The figure shows three views and two pictorial views of one solid part (mm, origin at its lowest corner). Answer the questions. Round coordinates to 2 decimals unless told otherwise and drop trailing zeros. Order: outer loops, then holes, each group sorted by start corner. A loop starts at its lowest first (then second) coordinate and runs counter-clockwise, first axis right, second up. Notation, with made-up numbers: (77.25, 56) -> (82.25, 56) arc R21 ccw to (82.25, 63) -> close; hole circle Ø1 at (-0.5, -0.75). An arc over 180 degrees is marked (long way). Return JSON: item names as keys, results as strings. Group by question number.
(1) The part is cut by section A-A (y = 2). Determine the outline of the cut face in (x, z).
(2) Determine the mould class of the marked faces 1, 2 and 3 for opening direction X: +X half, -X half, draft (parallel to the pull), parting line (faces both ways), or undercut.
(3) Each of these flat-tipped pins is pushed along its axis until it touches: pin 1 (4 mm diameter, centred on x = 17, z = 12, fed in from -Y); pin 2 (4 mm diameter, centred on y = 3, z = 13, fed in from +X). Where does it stop, or does it pass through?
(4) The part is cut by section C-C (z = 13.5). Determine the outline of the cut face in (x, y).
(5) The part is cut by section B-B (x = 50). Determine the outline of the cut face in (y, z) (1 decimal), plus the area to 3 significant figures.
(6) Consider line 1 (X direction, y = 9.75, z = 7.62); line 2 (Z direction, x = 45.72, y = 9.25); line 3 (Z direction, x = 44.5, y = 1.5). Determine where each line is inside the solid, lowest interval first. Write a range as [from, to].
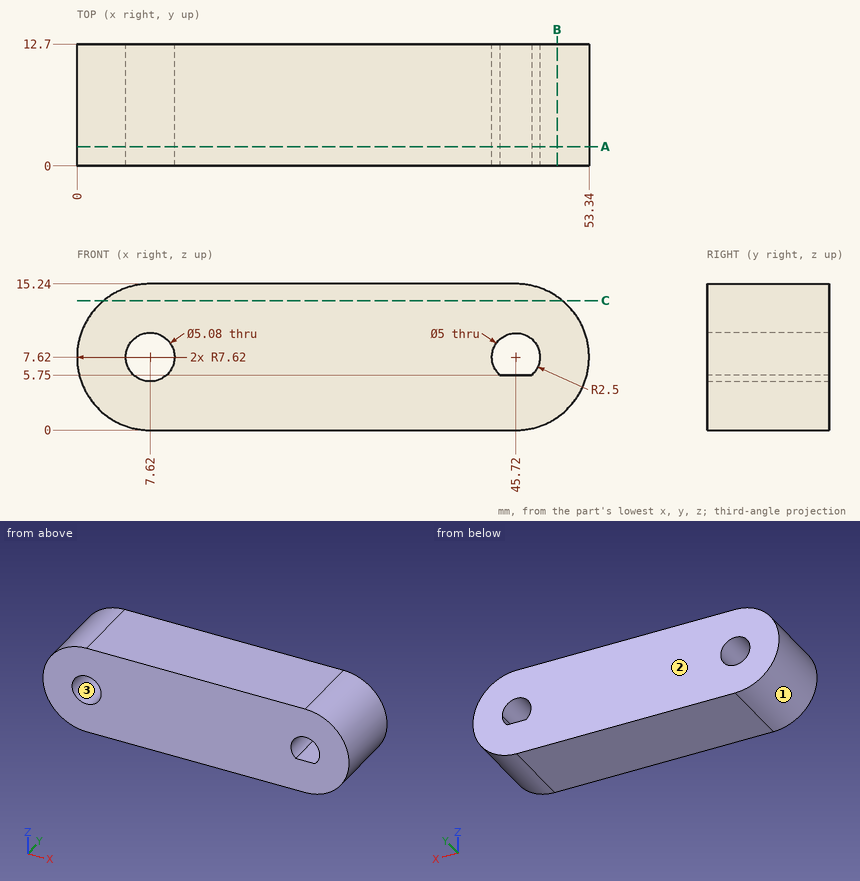
Answer below:
{
 "1": {"outline": "(7.62, 0) -> (45.72, 0) arc R7.62 ccw to (45.72, 15.24) -> (7.62, 15.24) arc R7.62 ccw to start; hole circle Ø5.08 at (7.62, 7.62); hole (44.06, 5.75) -> (47.38, 5.75) arc R2.5 ccw (long way) to start"},
 "2": {"face 1": "-X half", "face 2": "draft", "face 3": "undercut"},
 "3": {"pin 1": "stops at y = 0", "pin 2": "stops at x = 52.55"},
 "4": {"outline": "(2.77, 0) -> (50.57, 0) -> (50.57, 12.7) -> (2.77, 12.7) -> close"},
 "5": {"outline": "(0, 1.3) -> (12.7, 1.3) -> (12.7, 13.9) -> (0, 13.9) -> close", "area": "160 mm²"},
 "6": {"line 1": "x = [0, 5.08], [10.16, 43.22], [48.22, 53.34]", "line 2": "z = [0, 5.75], [10.12, 15.24]", "line 3": "z = [0, 5.75], [9.8, 15.24]"}
}
